from build123d import *

# Parameters (mm, degrees)
CROQUIS1_R              = 20
SALIENTE_EXTRUIR2_DEPTH = 18.5
CROQUIS3_R              = 25
SALIENTE_EXTRUIR3_DEPTH = 20
CROQUIS4_R              = 15.875
SALIENTE_EXTRUIR4_DEPTH = 15


with BuildPart() as part:
    # Croquis1 → Saliente-Extruir2 (new, symmetric)
    with BuildSketch(Plane.XY):
        Circle(CROQUIS1_R)
    extrude(amount=SALIENTE_EXTRUIR2_DEPTH, both=True)

    # Croquis3 → Saliente-Extruir3 (add)
    with BuildSketch(Plane.XY.offset(18.5)):
        Circle(CROQUIS3_R)
    extrude(amount=SALIENTE_EXTRUIR3_DEPTH)

    # Croquis4 → Saliente-Extruir4 (add)
    with BuildSketch(Plane.XY.offset(38.5)):
        Circle(CROQUIS4_R)
    extrude(amount=SALIENTE_EXTRUIR4_DEPTH)


solid = part.part
Could you check a few things on this model? Use its own coordinates, in mm. A direction names the side the tool comes from. Give positions to 0.01 mm unless a question says otherwise; leave off trailing zeros. Loops run counter-clockwise (first coordinate to the right, second up) from the corner with the lowest first, then second, coordinate; pieces in that order, holes last. Notation, with made-up numbers: (49.25, 78) -> (89.25, 78) arc R20 cw to (89.25, 99) -> close; hole circle Ø2 at (2.25, 51). An arc over 180 degrees is marked (long way). Return JSON: item names as keys, results as strings.
Item 1: If we section it at A-A on x = 8: List the corners of the cut face in (y, z) for me, plus the area to 3 significant figures.
Geometry results:
{"outline": "(-23.69, 18.5) -> (-18.33, 18.5) -> (-18.33, -18.5) -> (18.33, -18.5) -> (18.33, 18.5) -> (23.69, 18.5) -> (23.69, 38.5) -> (13.71, 38.5) -> (13.71, 53.5) -> (-13.71, 53.5) -> (-13.71, 38.5) -> (-23.69, 38.5) -> close", "area": "2,720 mm²"}
Item 2: I'm going to push flat-ended pins straight in: pin 1 (5 mm diameter, centred on y = -2, z = 36, fed in from +X); pin 2 (12 mm diameter, centred on y = 2.5, z = 4, fed in from -X); pin 3 (4 mm diameter, centred on x = -2, z = 23, fed in from -Y); pin 4 (3 mm diameter, centred on y = -17, z = 33, fed in from -X). Where does each tip first touch, or does it pass through?
Geometry results:
{"pin 1": "stops at x = 25", "pin 2": "stops at x = -20", "pin 3": "stops at y = -25", "pin 4": "stops at x = -19.62"}
Item 3: If we section it at D-D on y = -17.5: List the corners of the cut face in (x, z) for me.
Geometry results:
{"outline": "(-17.85, 18.5) -> (-9.68, 18.5) -> (-9.68, -18.5) -> (9.68, -18.5) -> (9.68, 18.5) -> (17.85, 18.5) -> (17.85, 38.5) -> (-17.85, 38.5) -> close"}
Item 4: Which directions (+Z, -Z, +X, -X, +Y, -Y) give clear straight access to the entire face, cutting with the end or side of a thin tool? Please do faces 1 (the cylindrical face through (-4.336, -19.524, 0.259)), 2 (the cylindrical face through (-3.441, -15.497, 45.895)), 3 (the flat face through (0, 0, 53.5)).
Geometry results:
{"face 1": "-Z", "face 2": "+Z", "face 3": "+Z, +X, -X, +Y, -Y"}
Item 5: If we section it at B-B on y = 0: List the corners of the cut face in (x, z) for me (3 decimals), plus the area to 3 significant figures.
Geometry results:
{"outline": "(-25, 18.5) -> (-20, 18.5) -> (-20, -18.5) -> (20, -18.5) -> (20, 18.5) -> (25, 18.5) -> (25, 38.5) -> (15.875, 38.5) -> (15.875, 53.5) -> (-15.875, 53.5) -> (-15.875, 38.5) -> (-25, 38.5) -> close", "area": "2,960 mm²"}
Item 6: If we section it at C-C on z = -5.5: List the corners of the cut face in (x, y) for me, plus the area to 3 significant figures.
Geometry results:
{"outline": "circle Ø40 at (0, 0)", "area": "1,260 mm²"}
Item 7: I need wall thicknesses on L1, parallel to Z at x = -20.5, y = -7.5; L2, parallel to Z at x = 10, y = -15; L3, parallel to X at y = -8, z = -15. Which ranges of each line are inside material? Lowest first, please. Write a range as from..to.
Geometry results:
{"L1": "z = 18.5..38.5", "L2": "z = -18.5..38.5", "L3": "x = -18.33..18.33"}
